For this review, take the finished solid that the model builds, in its own axes (mm). Face numbers are marked on the shaded views. A direction names the side the tool comes from. Round coordinates to 2 decimals unless told otherwise and drop trailing zeros. Write each loop counter-clockwise with the first axis right and the second up, starting at its lowest first coordinate (ties: lowest second). Pieces come first, ordered by that corner, then holes. Notation, with made-up numbers: (77.25, -19.75) -> (122.25, -19.75) arc R4 ccw to (122.25, -15.75) -> close; hole circle Ø1 at (12, 69.25). An arc over 180 degrees is marked (long way). Answer in a Markdown table with one row per item.
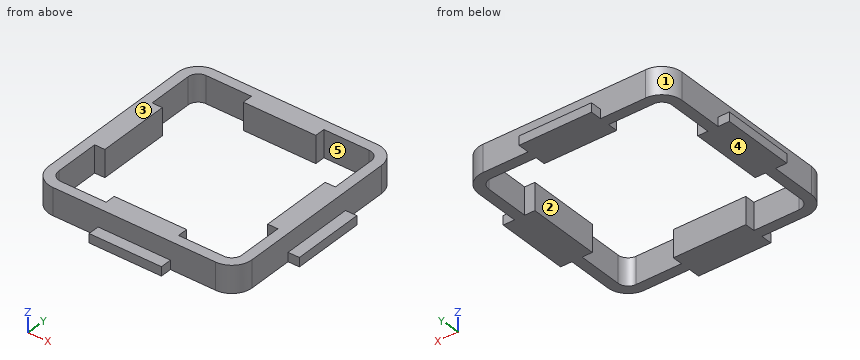
from build123d import *

# Parameters (mm, degrees)
F1_DEPTH = 15.24
F0_W     = 6.35
F0_H     = 20.32
F0_W_2   = 20.32
F0_H_2   = 6.35
F2_DEPTH = 5.08
F4_COUNT = 4


with BuildPart() as f1:
    # F0 (on Top) → F1 (new body)
    with BuildSketch(Plane.XY):
        with BuildLine():
            Line((0, 45.72), (0, 57.15))
            Line((0, 57.15), (-20.32, 57.15))
            Line((-20.32, 57.15), (-45.72, 57.15))
            ThreePointArc((-45.72, 57.15), (-53.802231, 53.802231), (-57.15, 45.72))
            Line((-57.15, 45.72), (-57.15, 20.32))
            Line((-57.15, 20.32), (-51.435, 20.32))
            Line((-51.435, 20.32), (-51.435, 45.759741))
            ThreePointArc((-51.435, 45.759741), (-49.758688, 49.78683), (-45.72, 51.435))
            Line((-45.72, 51.435), (-20.32, 51.435))
            Line((-20.32, 51.435), (-20.32, 45.72))
            Line((-20.32, 45.72), (0, 45.72))
        make_face()
        Polygon((-51.435, 20.32), (-57.15, 20.32), (-57.15, 0), (-45.72, 0), (-45.72, 20.32), align=None)
    extrude(amount=F1_DEPTH)

    # F0 (on Top) → F2 (join)
    with BuildSketch(Plane.XY):
        with Locations((-60.325, 10.16)):
            Rectangle(F0_W, F0_H)
        with Locations((-10.16, 60.325)):
            Rectangle(F0_W_2, F0_H_2)
    extrude(amount=F2_DEPTH)

    # F4: F1 ×4 about axis
    f4_axis = Axis((0, 0, 51.399533), (0, 0, -1))


with BuildPart() as f1_1:
    add(f1.part)
    for i in range(1, F4_COUNT):
        add(f1.part.rotate(f4_axis, i * 360 / F4_COUNT))


solid = f1_1.part
1) Clearance check with flat-ended pins moving along their axes: pin 1 Ø3 at (y, z) = (-11, 11) entering from -X; pin 2 Ø4.5 at (x, z) = (48.5, 8.5) entering from +Y; pin 3 Ø1 at (x, y) = (0, -45) entering from +Z; pin 4 Ø4 at (y, z) = (-37.5, 13) entering from +X. State where each tip first meets the part, or that it passes through.
Solved:
| item | result |
|---|---|
| pin 1 | x = -57.15 |
| pin 2 | y = 57.14 |
| pin 3 | through |
| pin 4 | x = 57.15 |
2) For the marked faces 4 and 5, list the 3-axis set-ups (+Z, -Z, +X, -X, +Y, -Y) from which the entire face can be reached by the end or side of a thin tool; tool diameter is ignored.
Solved:
| item | result |
|---|---|
| face 4 | -Z, +X, -X, +Y, -Y |
| face 5 | +Z, -Z |
3) Consider section A-A on x = -22. State the section outline as (y, z) points (3 decimals), then the cut area to 3 significant figures.
Solved:
| item | result |
|---|---|
| outline | (-57.15, 0) -> (-51.435, 0) -> (-51.435, 15.24) -> (-57.15, 15.24) -> close; (51.435, 0) -> (57.15, 0) -> (57.15, 15.24) -> (51.435, 15.24) -> close |
| area | 174 mm² |
4) For line 1 (X direction, y = 0, z = 13); line 2 (Y direction, x = 9.5, z = 1.5); line 3 (X direction, y = -21, z = 10) (3 decimals), list the stretches that pass through material, from the lowest coordinate up. Write a range as [from, to].
Solved:
| item | result |
|---|---|
| line 1 | [-57.15, -45.72], [45.72, 57.15] |
| line 2 | [-63.5, -45.72], [45.72, 63.5] |
| line 3 | [-57.15, -51.435], [51.435, 57.15] |
5) Consider section D-D on y = 17.5. State the section outline as (x, z) points, then the cut area to 3 significant figures.
Solved:
| item | result |
|---|---|
| outline | (-63.5, 0) -> (-45.72, 0) -> (-45.72, 15.24) -> (-57.15, 15.24) -> (-57.15, 5.08) -> (-63.5, 5.08) -> close; (45.72, 0) -> (63.5, 0) -> (63.5, 5.08) -> (57.15, 5.08) -> (57.15, 15.24) -> (45.72, 15.24) -> close |
| area | 413 mm² |
6) Mouldability with a two-part tool opening along X and no side actions: class the marked faces 1, 2 and 3 as pulls with the +X half, pulls with the -X half, needs draft (parallel to the pull), parting line crosses it, or undercut.
Solved:
| item | result |
|---|---|
| face 1 | pulls with the -X half |
| face 2 | undercut |
| face 3 | needs draft |
